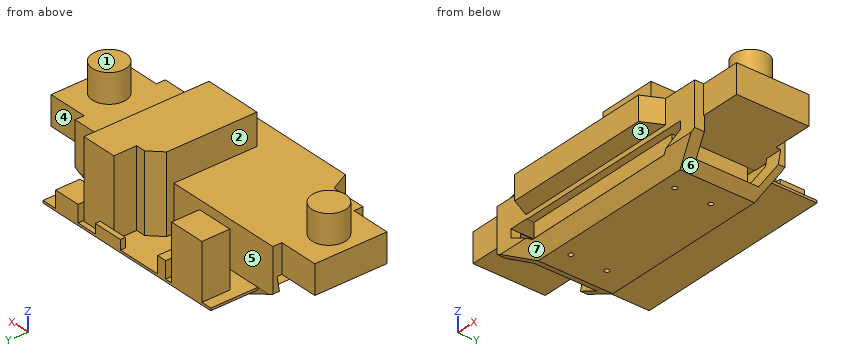
```python
from build123d import *
from OCP.BRepFilletAPI import BRepFilletAPI_MakeChamfer

# Parameters (mm, degrees)
BOSS_EXTRUDE1_DEPTH = 25
SKETCH2_W           = 84
SKETCH2_H           = 19.546511152
BOSS_EXTRUDE2_DEPTH = 24
SKETCH3_W           = 12
SKETCH3_H           = 30
BOSS_EXTRUDE3_DEPTH = 16.5
SKETCH4_W           = 12
SKETCH4_H           = 30
BOSS_EXTRUDE4_DEPTH = 16.5
SKETCH5_W           = 24
SKETCH5_H           = 52
BOSS_EXTRUDE5_DEPTH = 13
SKETCH9_W           = 70
SKETCH9_H           = 10
BOSS_EXTRUDE6_DEPTH = 8
CHAMFER1_SIZE       = 8
CHAMFER1_SIZE_2     = 4
SKETCH10_R          = 7
BOSS_EXTRUDE7_DEPTH = 12
SKETCH11_R          = 1
CUT_EXTRUDE1_DEPTH  = 5
CUT_EXTRUDE24_DEPTH = 37.4999
CUT_EXTRUDE25_REACH = 90.714
CUT_EXTRUDE26_DEPTH = 99
CUT_EXTRUDE27_REACH = 129.479
CUT_EXTRUDE28_DEPTH = 69.00303493
CUT_EXTRUDE29_REACH = 129.479
SKETCH19_W          = 69.00303493
SKETCH19_H          = 6
CUT_EXTRUDE30_DEPTH = 3
CUT_EXTRUDE32_DEPTH = 23
SKETCH21_W          = 3.997604332
SKETCH21_H          = 8.279085248
SKETCH21_W_2        = 11.293242608
SKETCH21_H_2        = 10.138766403
CUT_EXTRUDE33_DEPTH = 16
SKETCH22_W          = 12.573143588
SKETCH22_H          = 2.046511152
CUT_EXTRUDE34_DEPTH = 19
CUT_EXTRUDE35_DEPTH = 32


with BuildPart() as part:
    # Sketch1 → Boss-Extrude1 (new body)
    with BuildSketch(Plane.XY):
        Polygon((49.5, 0), (49.5, 18.75), (-49.5, 18.75), (-49.5, -18.75), (49.5, -18.75), align=None)
    extrude(amount=BOSS_EXTRUDE1_DEPTH)

    # Sketch2 → Boss-Extrude2 (add)
    with BuildSketch(Plane(origin=(0, 0, 5), x_dir=(-1, 0, 0), z_dir=(0, 0, -1))):
        with Locations((0, 28.523255576)):
            Rectangle(SKETCH2_W, SKETCH2_H)
    extrude(amount=-BOSS_EXTRUDE2_DEPTH)

    # Sketch3 → Boss-Extrude3 (add)
    with BuildSketch(Plane(origin=(49.5, 0, 0), x_dir=(0, 0, -1), z_dir=(1, 0, 0))):
        with Locations((-19, 0)):
            Rectangle(SKETCH3_W, SKETCH3_H)
    extrude(amount=BOSS_EXTRUDE3_DEPTH)

    # Sketch4 → Boss-Extrude4 (add)
    with BuildSketch(Plane.ZY.offset(49.5)):
        with Locations((19, 0)):
            Rectangle(SKETCH4_W, SKETCH4_H)
    extrude(amount=BOSS_EXTRUDE4_DEPTH)

    # Sketch5 → Boss-Extrude5 (add)
    with BuildSketch(Plane.XY.offset(25)):
        with Locations((12, 10.25)):
            Rectangle(SKETCH5_W, SKETCH5_H)
    extrude(amount=BOSS_EXTRUDE5_DEPTH)

    # Sketch9 → Boss-Extrude6 (add)
    with BuildSketch(Plane.XZ.offset(18.75)):
        with Locations((0, 20)):
            Rectangle(SKETCH9_W, SKETCH9_H)
    extrude(amount=BOSS_EXTRUDE6_DEPTH)

    # Chamfer1
    chamfer1_edges_1 = [part.edges().sort_by_distance(p)[0] for p in [
        (-35, -26.75, 20),
    ]]
    chamfer1_side_1 = [part.faces().sort_by_distance(p)[0] for p in [
        (-35, -26.67, 20),
    ]]
    chamfer1_edges_2 = [part.edges().sort_by_distance(p)[0] for p in [
        (35, -26.75, 20),
    ]]
    chamfer1_side_2 = [part.faces().sort_by_distance(p)[0] for p in [
        (35, -26.67, 20),
    ]]
    chamfer1 = BRepFilletAPI_MakeChamfer(part.part.solid().wrapped)
    for e in chamfer1_edges_1:
        chamfer1.Add(CHAMFER1_SIZE - 0.0001, CHAMFER1_SIZE_2 - 0.0001, e.wrapped, chamfer1_side_1[0].wrapped)
    for e in chamfer1_edges_2:
        chamfer1.Add(CHAMFER1_SIZE - 0.0001, CHAMFER1_SIZE_2 - 0.0001, e.wrapped, chamfer1_side_2[0].wrapped)
    add(Compound.cast(chamfer1.Shape()), mode=Mode.REPLACE)  # a hair under: the kernel refuses the full size

    # Sketch10 → Boss-Extrude7 (add)
    with BuildSketch(Plane.XY.offset(25)):
        with Locations((-55, 0)):
            Circle(SKETCH10_R)
        with Locations((55, 0)):
            Circle(SKETCH10_R)
    extrude(amount=BOSS_EXTRUDE7_DEPTH)

    # Sketch11 → Cut-Extrude1 (cut)
    with BuildSketch(Plane(origin=(0, 0, 0), x_dir=(-1, 0, 0), z_dir=(0, 0, -1))):
        with Locations((-26, 7.5)):
            Circle(SKETCH11_R)
        with Locations((26, 7.5)):
            Circle(SKETCH11_R)
        with Locations((26, -7.5)):
            Circle(SKETCH11_R)
        with Locations((-26, -7.5)):
            Circle(SKETCH11_R)
    extrude(amount=-CUT_EXTRUDE1_DEPTH, mode=Mode.SUBTRACT)

    # Sketch12 → Cut-Extrude24 (cut)
    with BuildSketch(Plane.XZ.offset(18.75)):
        Polygon((49.5, 7), (35.5, 0), (49.5, 0), align=None)
        Polygon((-49.5, 0), (-49.5, 7), (-35.5, 0), align=None)
        Polygon((-42.50303493, 13.206106321), (-42.50303493, 9.79786642), (-32.90730209, 5), (32.904267164, 5), (42.5, 9.797866418), (42.5, 13), (34.5, 13), (34.5, 7), (-34.50303493, 7), (-34.50303493, 13.206106321), align=None)
    extrude(amount=-CUT_EXTRUDE24_DEPTH, mode=Mode.SUBTRACT)

    # Sketch13 → Cut-Extrude25 (cut, up to next)
    with BuildSketch(Plane.XZ.offset(-18.7499), mode=Mode.PRIVATE) as cut_extrude25_sk1:
        Polygon((49.5, 7), (49.5, 0), (35.5, 0), align=None)
    cut_extrude25_tool1 = extrude(cut_extrude25_sk1.sketch, amount=-CUT_EXTRUDE25_REACH, mode=Mode.PRIVATE) & part.part
    # Sketch13 → Cut-Extrude25 (cut, up to next)
    with BuildSketch(Plane.XZ.offset(-18.7499), mode=Mode.PRIVATE) as cut_extrude25_sk2:
        Polygon((-35.5, 0), (-49.5, 0), (-49.5, 7), align=None)
    cut_extrude25_tool2 = extrude(cut_extrude25_sk2.sketch, amount=-CUT_EXTRUDE25_REACH, mode=Mode.PRIVATE) & part.part
    add(cut_extrude25_tool1.solids().sort_by_distance((44.833333, 18.7499, 2.333333))[0], mode=Mode.SUBTRACT)
    add(cut_extrude25_tool2.solids().sort_by_distance((-44.833333, 18.7499, 2.333333))[0], mode=Mode.SUBTRACT)

    # Sketch14 → Cut-Extrude26 (cut)
    with BuildSketch(Plane.ZY.offset(49.5)):
        Polygon((13, 15.669938024), (7, 15.669938024), (7, -14.75), (2.533243234, -10.75), (2.533243234, 15.25), (13, 16.991870924), align=None)
        Polygon((0, 17.75), (0, 18.75), (6.008916401, 18.75), align=None)
        Polygon((0, -13.25), (6.141790553, -18.75), (0, -18.75), align=None)
    extrude(amount=-CUT_EXTRUDE26_DEPTH, mode=Mode.SUBTRACT)

    # Sketch15 → Cut-Extrude27 (cut, up to next)
    with BuildSketch(Plane.ZY.offset(49.5), mode=Mode.PRIVATE) as cut_extrude27_sk1:
        Polygon((7, -14.75), (13, -14.75), (13, 15), (13, 15.669938024), (7, 15.669938024), align=None)
    cut_extrude27_tool1 = extrude(cut_extrude27_sk1.sketch, amount=-CUT_EXTRUDE27_REACH, mode=Mode.PRIVATE) & part.part
    add(cut_extrude27_tool1.solids().sort_by_distance((-49.5, 0.459969, 10))[0], mode=Mode.SUBTRACT)

    # Sketch16 → Cut-Extrude28 (cut)
    with BuildSketch(Plane.ZY.offset(34.50303493)):
        Polygon((13, 15.669938024), (13.206106321, 15.669938024), (13.206106321, 18.7499), (7, 18.7499), (7, 15.993354786), (13, 16.991870924), align=None)
    extrude(amount=-CUT_EXTRUDE28_DEPTH, mode=Mode.SUBTRACT)

    # Sketch18 → Cut-Extrude29 (cut, up to next)
    with BuildSketch(Plane(origin=(49.5, 0, 0), x_dir=(0, 0, -1), z_dir=(1, 0, 0)), mode=Mode.PRIVATE) as cut_extrude29_sk1:
        Polygon((-13, 15.669938024), (-13, 15), (-13, -14.75), (-7, -14.75), (-7, 15.669938024), align=None)
    cut_extrude29_tool1 = extrude(cut_extrude29_sk1.sketch, amount=-CUT_EXTRUDE29_REACH, mode=Mode.PRIVATE) & part.part
    add(cut_extrude29_tool1.solids().sort_by_distance((49.5, 0.459969, 10))[0], mode=Mode.SUBTRACT)

    # Sketch19 → Cut-Extrude30 (cut)
    with BuildSketch(Plane.XZ.offset(18.75)):
        with Locations((-0.001517465, 10)):
            Rectangle(SKETCH19_W, SKETCH19_H)
    extrude(amount=-CUT_EXTRUDE30_DEPTH, mode=Mode.SUBTRACT)

    # Sketch20 → Cut-Extrude32 (cut)
    with BuildSketch(Plane.XY.offset(29)):
        Polygon((3.229837256, 36.25), (0, 36.25), (0, 18.75), (-42, 18.75), (-42, 38.296511152), (-37.533682083, 38.296511152), (-37.533682083, 26.659686261), (-22.363703257, 26.659686261), (-22.363703257, 38.296511152), (-19.429087816, 38.296511152), (-19.429087816, 30.017425904), (-15.431483484, 30.017425904), (-15.431483484, 38.296511152), (3.229837256, 38.296511152), align=None)
        Polygon((24.40253089, 38.296511152), (24.40253089, 28.157744749), (35.695773498, 28.157744749), (35.695773498, 38.296511152), (42, 38.296511152), (42, 18.75), (24, 18.75), (24, 36.25), (15.802980844, 36.25), (15.802980844, 38.296511152), align=None)
    extrude(amount=-CUT_EXTRUDE32_DEPTH, mode=Mode.SUBTRACT)

    # Sketch21 → Cut-Extrude33 (cut)
    with BuildSketch(Plane.XY.offset(29)):
        with Locations((-17.43028565, 34.156968528)):
            Rectangle(SKETCH21_W, SKETCH21_H)
        with Locations((30.049152194, 33.227127951)):
            Rectangle(SKETCH21_W_2, SKETCH21_H_2)
    extrude(amount=-CUT_EXTRUDE33_DEPTH, mode=Mode.SUBTRACT)

    # Sketch22 → Cut-Extrude34 (cut)
    with BuildSketch(Plane.XY.offset(29)):
        with Locations((9.51640905, 37.273255576)):
            Rectangle(SKETCH22_W, SKETCH22_H)
    extrude(amount=-CUT_EXTRUDE34_DEPTH, mode=Mode.SUBTRACT)

    # Sketch23 → Cut-Extrude35 (cut)
    with BuildSketch(Plane.XY.offset(38)):
        Polygon((0, 21.75), (5, 26.75), (9, 26.75), (9, 36.25), (0, 36.25), align=None)
    extrude(amount=-CUT_EXTRUDE35_DEPTH, mode=Mode.SUBTRACT)


solid = part.part
```
Read the model definition and answer for the solid it produces. Units are mm, in the model's axes. Face numbers are marked on the shaded views. A direction names the side the tool comes from. Coordinates: 2 decimals unless noted, no trailing zeros. Write each loop counter-clockwise with the first axis right and the second up, starting at its lowest first coordinate (ties: lowest second). Pieces come first, ordered by that corner, then holes. Notation, with made-up numbers: (54, 77) -> (94, 77) arc R14 cw to (94, 92) -> close; hole circle Ø6 at (1.5, 16). An arc over 180 degrees is marked (long way). Return JSON: item names as keys, results as strings.
1. Find the intervals of material crossed by line 1 along Z through (x, y) = (28, 3); line 2 along Z through (x, y) = (21.5, 16); line 3 along X through (y, z) = (7, 1), in increasing order. Write a range as from..to.
Found:
{"line 1": "0..2.53, 7..25", "line 2": "0..5, 13.21..38", "line 3": "-37.5..-26.87, -25.13..25.13, 26.87..37.5"}
2. A tool of negligible diameter and unlimited length cuts with its end or side. For the marked faces 1, 2 and 3, from which of +Z, -Z, +X, -X, +Y, -Y can it reach the whole face along a straight path? Write none if from no direction.
Found:
{"face 1": "+Z, +X, +Y, -Y", "face 2": "+Z, +Y", "face 3": "-Z, +X, -X, -Y"}
3. A cutting plane is placed at C-C (y = 24). Determine the outline of the cut face in (x, z), and give its area (3 significant figures).
Found:
{"outline": "(-42, 5) -> (42, 5) -> (42, 6) -> (24, 6) -> (24, 38) -> (2.25, 38) -> (2.25, 6) -> (-42, 6) -> close", "area": "780 mm2"}
4. Determine the mould class of the marked faces 4, 5, 6 and 7 for opening direction Y: pulls with the +Y half, pulls with the -Y half, needs draft (parallel to the pull), parting line crosses it, or undercut.
Found:
{"face 4": "pulls with the +Y half", "face 5": "undercut", "face 6": "needs draft", "face 7": "pulls with the -Y half"}
5. A cutting plane is placed at D-D (x = -55). Determine the outline of the cut face in (y, z), and give its area (3 significant figures).
Found:
{"outline": "(-15, 13) -> (15, 13) -> (15, 25) -> (7, 25) -> (7, 37) -> (-7, 37) -> (-7, 25) -> (-15, 25) -> close", "area": "528 mm2"}
6. Each of these flat-tipped pins is pushed along its axis until it touches: P1, Ø4, axis at x = -52, z = 11.5, coming from the +Y side; P2, Ø8, axis at y = 22, z = 9, coming from the +X side; P3, Ø3, axis at y = 27.5, z = 34, coming from the +X side. Where does it stop, or does it pass through?
Found:
{"P1": "y = 15", "P2": "x = 49.5", "P3": "x = 24"}
7. A cutting plane is placed at B-B (y = 0). Determine the outline of the cut face in (x, z).
Found:
{"outline": "(-66, 13) -> (-42.5, 13) -> (-42.5, 13.21) -> (-34.5, 13.21) -> (-34.5, 7) -> (34.5, 7) -> (34.5, 13) -> (66, 13) -> (66, 25) -> (62, 25) -> (62, 37) -> (48, 37) -> (48, 25) -> (24, 25) -> (24, 38) -> (0, 38) -> (0, 25) -> (-48, 25) -> (-48, 37) -> (-62, 37) -> (-62, 25) -> (-66, 25) -> close; (-40.57, 2.53) -> (-35.5, 0) -> (35.5, 0) -> (40.57, 2.53) -> close"}
8. A cutting plane is placed at A-A (x = -14). Give the number of separate pieces and of enclosed holes in the cut face, and give its area (3 significant figures).
Found:
{"separate pieces": "3", "enclosed holes": "0", "area": "838 mm2"}
